Could you check a few things on this drawing? It's one solid part, dimensions in mm from its lowest x, y, z. Round coordinates to 2 decimals unless told otherwise and drop trailing zeros. Write each loop counter-clockwise with the first axis right and the second up, starting at its lowest first coordinate (ties: lowest second). Pieces come first, ordered by that corner, then holes. Notation, with made-up numbers: (-31, 81.5) - (21, 81.5) arc R29 cw to (21, 105.5) - close; hole circle Ø6 at (73.5, 18). An arc over 180 degrees is marked (long way). Write item = value, one per line. Start each with the question number.
Item 1: If we section it at D-D (x = 31.5): Please give me the cut outline in (y, z) (1 decimal), and give its area (3 significant figures).
Item 2: If I drill on line 1 along Z through (x, y) = (32, 21) (1 decimal); line 2 along X through (y, z) = (28.5, 2.05) (1 decimal); line 3 along Y through (x, z) = (19, 1.35) (1 decimal), over which ranges is the centre line in solid material (lowest first)? Write a range as [from, to].
Item 3: If we section it at C-C (z = 2.6): Give the number of separate pieces and of enclosed holes in the cut face, and give its area (3 significant figures).
Item 4: If we section it at B-B (y = 24.5): Please give me the cut outline in (x, z) (1 decimal).
Item 5: For P1, Ø3, axis at x = 31, y = 24.5, coming from the +Z side; P2, Ø3, axis at x = 4.76, y = 20.64, coming from the +Z side; P3, Ø2, axis at x = 6.5, z = 3.5, coming from the -Y side; P4, Ø22, axis at x = 20.64, y = 20.64, coming from the +Z side (1 decimal), each with a flat end and sliding along its axis, tell me the tip position at first contact or that it passes through.
Item 6: If we section it at A-A (x = 26): Please give me the cut outline in (y, z) (1 decimal).
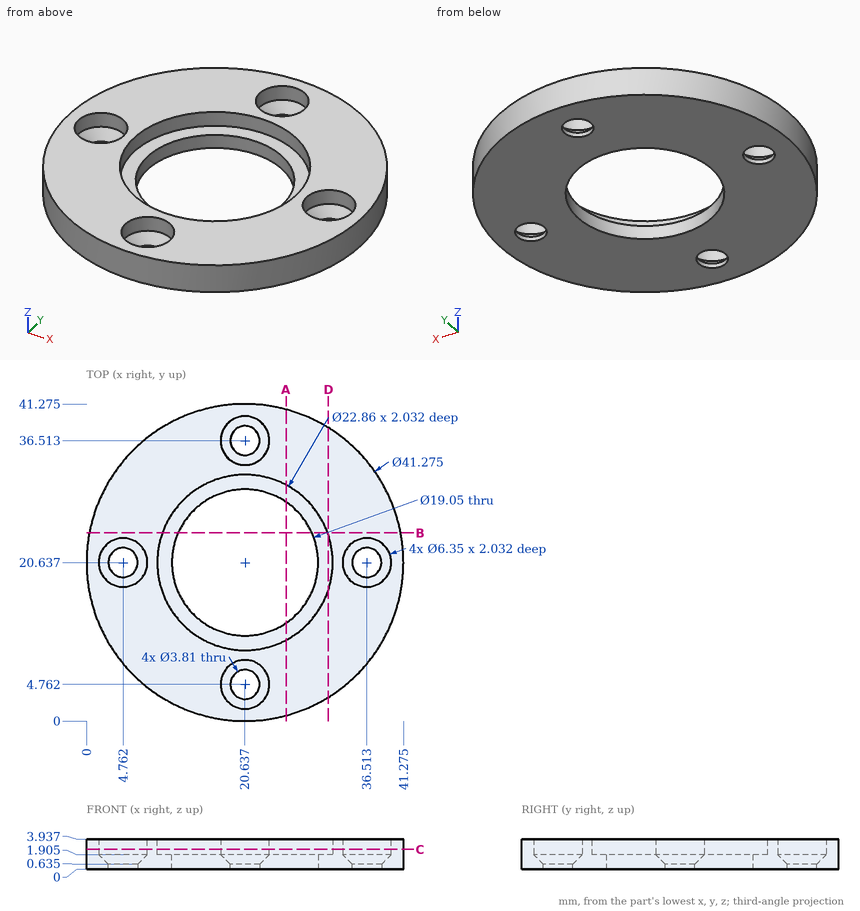
Reply:
q1.outline = (3.1, 0) - (38.2, 0) - (38.2, 3.9) - (24.2, 3.9) - (24.2, 1.9) - (17.1, 1.9) - (17.1, 3.9) - (3.1, 3.9) - close
q1.area = 124 mm2
q2.line_1 = [0, 1.9]
q2.line_2 = [1.6, 12.3], [28.9, 39.7]
q2.line_3 = [0.1, 2.7], [6.8, 11.3], [30, 34.5], [38.6, 41.2]
q3.separate_pieces = 1
q3.enclosed_holes = 5
q3.area = 801 mm2
q4.outline = (0.4, 0) - (11.9, 0) - (11.9, 1.9) - (9.9, 1.9) - (9.9, 3.9) - (0.4, 3.9) - close; (29.3, 0) - (40.9, 0) - (40.9, 3.9) - (31.4, 3.9) - (31.4, 1.9) - (29.3, 1.9) - close
q5.P1 = 3.94
q5.P2 = through
q5.P3 = 4.72
q5.P4 = 1.9
q6.outline = (0.7, 0) - (12.8, 0) - (12.8, 1.9) - (10.5, 1.9) - (10.5, 3.9) - (0.7, 3.9) - close; (28.5, 0) - (40.6, 0) - (40.6, 3.9) - (30.7, 3.9) - (30.7, 1.9) - (28.5, 1.9) - close
